Source: CAD feature listing. Evaluate the final solid. Frame: model axes, mm. Give positions to 0.01 mm unless a question says otherwise; leave off trailing zeros. Order: outer loops, then holes, each group sorted by start corner. A loop starts at its lowest first (then second) coordinate and runs counter-clockwise, first axis right, second up. Notation, with made-up numbers: M -4.75,25.25 L 27.25,25.25 A28 ccw 27.25,55.25 Z; hole C 73,-25 d7. An arc over 180 degrees is marked long. Answer as a JSON object with one key per item and string values. Group by question number.
1. Material intervals for L1, parallel to X at y = 5.1, z = -250.5; L2, parallel to Y at x = -0.4, z = -208; L3, parallel to Z at x = -0.1, y = 1.8, sorted ascending. Write a range as [from, to].
2. Section query B-B (z = -202.5). Output: boundary loops of the cut face in (x, y), plus the area to 3 significant figures.
3. Section query C-C (y = 2.55). Output: boundary loops of the cut face in (x, z).
4. Section query A-A (x = 0). Output: boundary loops of the cut face in (y, z), plus the area to 3 significant figures.
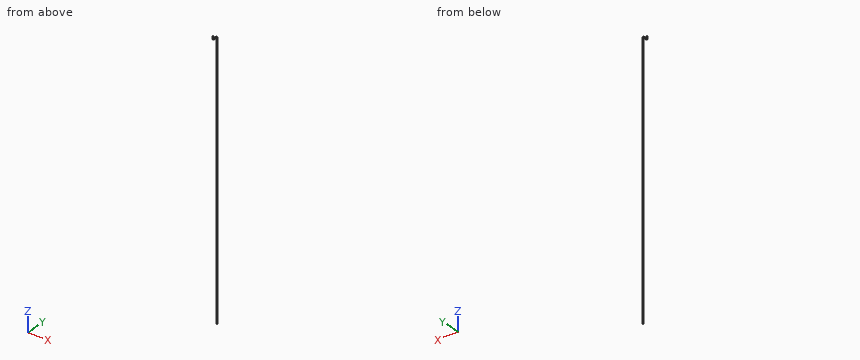
Autodesk Inventor part; units mm, degrees
ref_plane "YZ Plane" through (0, 0, 0) normal (1, 0, 0) x (0, 1, 0)
ref_plane "XZ Plane" through (0, 0, 0) normal (0, 1, 0) x (-1, 0, 0)
ref_plane "XY Plane" through (0, 0, 0) normal (0, 0, 1) x (1, 0, 0)
sketch "Sketch1" plane through (0, 0, 0) normal (0, 0, 1) x (1, 0, 0)
  circle A0 centre (0, 0) radius 0.5
  dimension "d0" = 1
sketch "Sketch2" plane through (0, 0, 0) normal (1, 0, 0) x (0, 1, 0)
  line L0 (0, 0) -> (0, -2)
  line L1 (1, -3) -> (4, -3)
  line L2 (5, -4) -> (5, -268)
  arc A0 (5, -4) -> (4, -3) centre (4, -4) ccw
  arc A1 (0, -2) -> (1, -3) centre (1, -2) ccw
  point P0 (0, -3)
  point P1 (5, -3)
  dimension "d1" = 3
  dimension "d2" = 5
  dimension "d3" = 265
  dimension "d4" = 1
sweep "Sweep1" add profiles "Sketch1" path "Sketch2"
chamfer "Chamfer1" distance 0.2 angle 45 6 edges at (-0.5, 0, 0) (-0.5, 0, -2) (-0.5, 1, -3) (-0.5, 4, -3) (-0.5, 5, -4) (-0.5, 5, -268)
equation "\"Length\" = 265"
properties part number "TAIL" material "Steel, High Strength, Low Alloy"
Answer sheet:
{
 "1": {"L1": "[-0.49, 0.49]", "L2": "[4.7, 5.3]", "L3": "[-3.49, -2.51]"},
 "2": {"outline": "C 0,5 d1", "area": "0.785 mm^2"},
 "3": {"outline": "C 0,-3 d1"},
 "4": {"outline": "M -0.5,-2 A1.5 ccw 1,-3.5 L 4,-3.5 A0.5 cw 4.5,-4 L 4.5,-267.8 L 4.7,-268 L 5.3,-268 L 5.5,-267.8 L 5.5,-4 A1.5 ccw 4,-2.5 L 1,-2.5 A0.5 cw 0.5,-2 L 0.5,-0.2 L 0.3,0 L -0.3,0 L -0.5,-0.2 Z", "area": "272 mm^2"}
}
